Part model, mm, in its own coordinate system. A direction names the side the tool comes from. Give positions to 0.01 mm unless a question says otherwise; leave off trailing zeros. Order: outer loops, then holes, each group sorted by start corner. A loop starts at its lowest first (then second) coordinate and runs counter-clockwise, first axis right, second up. Notation, with made-up numbers: M 56.25,88 L 79.25,88 A38 ccw 79.25,126 Z; hole C 67.5,60.25 d11. An arc over 180 degrees is marked long. Return JSON: item names as keys, results as strings.
from build123d import *

# Parameters (mm, degrees)
CHAMFER1_SIZE              = 0.254
CHAMFER1_EDGE_2_SIZE2      = 0.215388858
CHAMFER1_EDGE_2_SIZE       = 0.254
SKETCH4_R                  = 3.5
CUT_EXTRUDE1_DEPTH         = 2.5
M7X0_75_TAPPED_HOLE1_D     = 6
M7X0_75_TAPPED_HOLE1_DEPTH = 10.954004
M7X0_75_TAPPED_HOLE1_TIP   = 1.802581857


with BuildPart() as part:
    # Sketch1 → Revolve1 (revolve)
    with BuildSketch(Plane.XY):
        with BuildLine():
            Line((0, 25.4), (-4.80695, 25.4))
            Line((-4.80695, 25.4), (-3.8227, 30.2387))
            Line((-3.8227, 30.2387), (-5.588, 30.2387))
            Line((-5.588, 30.2387), (-5.588, 36.9824))
            Line((-5.588, 36.9824), (-1.563367534, 40.735379295))
            ThreePointArc((-1.563367534, 40.735379295), (-0.840141831, 41.19169557), (0, 41.3512))
            Line((0, 41.3512), (0, 25.4))
        make_face()
    revolve(axis=Axis((0, 25.4, 0), (0, 1, 0)))

    # Chamfer1
    chamfer1_edges = [part.edges().sort_by_distance(p)[0] for p in [
        (5.588, 30.2387, 0),
    ]]
    chamfer(chamfer1_edges, length=CHAMFER1_SIZE)

    # Chamfer1 edge 2
    chamfer1_edge_2_edges = [part.edges().sort_by_distance(p)[0] for p in [
        (4.80695, 25.4, 0),
    ]]
    chamfer(chamfer1_edge_2_edges, length=CHAMFER1_EDGE_2_SIZE, length2=CHAMFER1_EDGE_2_SIZE2)

    # Sketch4 → Cut-Extrude1 (cut)
    with BuildSketch(Plane.XZ.offset(-25.4)):
        Circle(SKETCH4_R)
    extrude(amount=-CUT_EXTRUDE1_DEPTH, mode=Mode.SUBTRACT)

    # M7x0.75 Tapped Hole1
    with Locations(Plane(origin=(0, 25.4, 0), x_dir=(-1, 0, 0), z_dir=(0, -1, 0))):
        with Locations((0, 0), (96.139395676, -180.684699687)):
            Hole(M7X0_75_TAPPED_HOLE1_D / 2, depth=M7X0_75_TAPPED_HOLE1_DEPTH)
            with Locations((0, 0, -(M7X0_75_TAPPED_HOLE1_DEPTH + M7X0_75_TAPPED_HOLE1_TIP / 2))):  # 118° drill point
                Cone(0, M7X0_75_TAPPED_HOLE1_D / 2, M7X0_75_TAPPED_HOLE1_TIP, mode=Mode.SUBTRACT)


solid = part.part
Q1. Band-saw the part on A-A (y = 33). Give the cut face in (x, z), then the cut area to 3 significant figures.
Established:
{"outline": "C 0,0 d11.18; hole C 0,0 d6", "area": "69.8 mm²"}
Q2. Two-plate mould, pull along Y, no slides. Class faces 4 (the conical face through (0.113, 37.844, 0.509)), 5 (the cylindrical face through (4.434, 33.783, -3.4)), 6 (the conical face through (1.4, 40.55, -1.07)), 7 (the flat face through (-4, 30.239, 1)): +Y half, -Y half, draft (parallel to the pull), parting line (faces both ways), or undercut.
Established:
{"face 4": "-Y half", "face 5": "draft", "face 6": "+Y half", "face 7": "undercut"}
Q3. Probe line 1 along Z through (x, y) = (0, 33.5); line 2 along Z through (x, y) = (0, 26.3); line 3 along X through (y, z) = (27.25, 1.75). List the from-to ranges inside material, lowest first.
Established:
{"line 1": "z = -5.59 to -3, 3 to 5.59", "line 2": "z = -4.62 to -3.5, 3.5 to 4.62", "line 3": "x = -4.07 to -3.03, 3.03 to 4.07"}
Q4. Band-saw the part on B-B (y = 27). Give the cut face in (x, z).
Established:
{"outline": "C 0,0 d8.96; hole C 0,0 d7"}
Q5. Pin check, flat tips, straight feed: pin 1 (6 mm diameter, centred on x = -3.5, z = -1.5, fed in from +Y); pin 2 (6 mm diameter, centred on y = 30, z = -3.5, fed in from -X). Stop position of each tip, or through.
Established:
{"pin 1": "stops at y = 41.2", "pin 2": "stops at x = -5.56"}
Q6. 3-axis set-ups, long thin cutter, end or side, ignore diameter. For faces 1 (the conical face through (3.234, 28.996, -2.48)), 2 (the flat face through (0, 25.4, -4)), 3 (the flat face through (3, 27.9, 1)): which of +Z, -Z, +X, -X, +Y, -Y reach the whole face in a straight line?
Established:
{"face 1": "none", "face 2": "+Z, -Z, +X, -X, -Y", "face 3": "-Y"}
